Part model, mm, in its own coordinate system. Face numbers are marked on the shaded views. Round coordinates to 2 decimals unless told otherwise and drop trailing zeros. Order: outer loops, then holes, each group sorted by start corner. A loop starts at its lowest first (then second) coordinate and runs counter-clockwise, first axis right, second up. Notation, with made-up numbers: (81.5, 35) - (89.5, 35) arc R18 ccw to (89.5, 60) - close; hole circle Ø2 at (21.5, 20). An arc over 180 degrees is marked (long way). Return JSON: item names as keys, results as strings. Group by question number.
Item 1: Saw through at C-C on x = 14. List the corners of the cut face in (y, z).
Item 2: Saw through at D-D on y = -0.25. List the corners of the cut face in (x, z).
Item 3: Probe probe 1 along Z at (x, y) = (13.5, 3.5); probe 2 along X at (y, z) = (0, 3.5); probe 3 along Y at (x, z) = (12.75, 7.5). List the from-to ranges inside material, lowest first.
Item 4: Drop flat-ended pins along their axis: pin 1 (2.5 mm diameter, centred on x = 13.47, z = 5, fed in from -Y); pin 2 (1 mm diameter, centred on x = 9.5, z = 15, fed in from -Y). Give the stop position or say it passes through.
Item 5: Saw through at A-A on z = 5. List the corners of the cut face in (x, y), and give its area (3 significant figures).
Item 6: Saw through at B-B on y = 1.5. List the corners of the cut face in (x, z), and give its area (3 significant figures).
Item 7: Two-plate mould, pull along X, no slides. Class the marked faces 1, 2 and 3: released by +X, released by -X, zero draft, split by the parting line, or undercut.
```python
from build123d import *

# Parameters (mm, degrees)
ESBO_O1_W                  = 12
ESBO_O1_H                  = 12
ESBO_O1_R                  = 1.7
RESSALTO_EXTRUS_O1_DEPTH   = 22
ESBO_O2_R                  = 1.5
CORTE_EXTRUS_O1_DEPTH      = 7
CORTE_EXTRUS_O1_DEPTH_BACK = 10
FILETE2_R                  = 3
FILETE3_R                  = 3
FILETE4_R                  = 3
FILETE5_R                  = 3


with BuildPart() as part:
    # Esboço1 → Ressalto-extrusão1 (new body)
    with BuildSketch(Plane.XY):
        with Locations((13.471698113, -0.79245283)):
            Rectangle(ESBO_O1_W, ESBO_O1_H)
        with Locations((13.471698113, -0.79245283)):
            Circle(ESBO_O1_R, mode=Mode.SUBTRACT)
    extrude(amount=RESSALTO_EXTRUS_O1_DEPTH)

    # Esboço2 → Corte-extrusão1 (cut, two sides)
    with BuildSketch(Plane(origin=(0, 0, 0), x_dir=(1, 0, 0), z_dir=(0, 1, 0))) as corte_extrus_o1_sk:
        with Locations((13.471698113, -5)):
            Circle(ESBO_O2_R)
    extrude(amount=CORTE_EXTRUS_O1_DEPTH, mode=Mode.SUBTRACT)
    extrude(corte_extrus_o1_sk.sketch, amount=-CORTE_EXTRUS_O1_DEPTH_BACK, mode=Mode.SUBTRACT)

    # Filete2
    filete2_edges = [part.edges().sort_by_distance(p)[0] for p in [
        (7.471698113, 5.20754717, 11),
    ]]
    fillet(filete2_edges, radius=FILETE2_R)

    # Filete3
    filete3_edges = [part.edges().sort_by_distance(p)[0] for p in [
        (7.471698113, -6.79245283, 11),
    ]]
    fillet(filete3_edges, radius=FILETE3_R)

    # Filete4
    filete4_edges = [part.edges().sort_by_distance(p)[0] for p in [
        (19.471698113, -6.79245283, 11),
    ]]
    fillet(filete4_edges, radius=FILETE4_R)

    # Filete5
    filete5_edges = [part.edges().sort_by_distance(p)[0] for p in [
        (19.471698113, 5.20754717, 11),
    ]]
    fillet(filete5_edges, radius=FILETE5_R)


solid = part.part
```
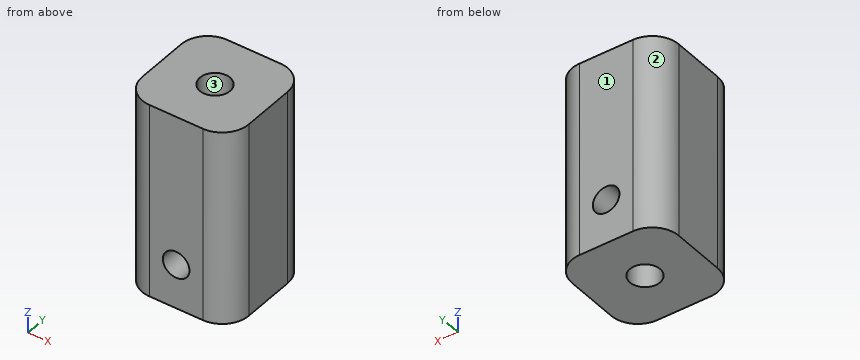
Filled in:
{
 "1": {"outline": "(-6.79, 0) - (-2.41, 0) - (-2.41, 3.6) - (-6.79, 3.6) - close; (-6.79, 6.4) - (-2.41, 6.4) - (-2.41, 22) - (-6.79, 22) - close; (0.82, 0) - (5.21, 0) - (5.21, 3.6) - (0.82, 3.6) - close; (0.82, 6.4) - (5.21, 6.4) - (5.21, 22) - (0.82, 22) - close"},
 "2": {"outline": "(7.47, 0) - (11.86, 0) - (11.86, 22) - (7.47, 22) - close; (15.08, 0) - (19.47, 0) - (19.47, 22) - (15.08, 22) - close"},
 "3": {"probe 1": "z = 0 to 3.5, 6.5 to 22", "probe 2": "x = 7.47 to 11.97, 14.98 to 19.47", "probe 3": "y = -6.79 to -2.33, 0.75 to 5.21"},
 "4": {"pin 1": "passes through", "pin 2": "stops at y = -6.76"},
 "5": {"outline": "(7.47, -3.79) arc R3 ccw to (10.47, -6.79) - (11.97, -6.79) - (11.97, -1.59) arc R1.7 cw to (11.97, 0.01) - (11.97, 5.21) - (10.47, 5.21) arc R3 ccw to (7.47, 2.21) - close; (14.97, -6.79) - (16.47, -6.79) arc R3 ccw to (19.47, -3.79) - (19.47, 2.21) arc R3 ccw to (16.47, 5.21) - (14.97, 5.21) - (14.97, 0.01) arc R1.7 cw to (14.97, -1.59) - close", "area": "99.8 mm^2"},
 "6": {"outline": "(7.47, 0) - (19.47, 0) - (19.47, 22) - (7.47, 22) - close; hole circle Ø3 at (13.47, 5)", "area": "257 mm^2"},
 "7": {"face 1": "zero draft", "face 2": "released by -X", "face 3": "undercut"}
}
